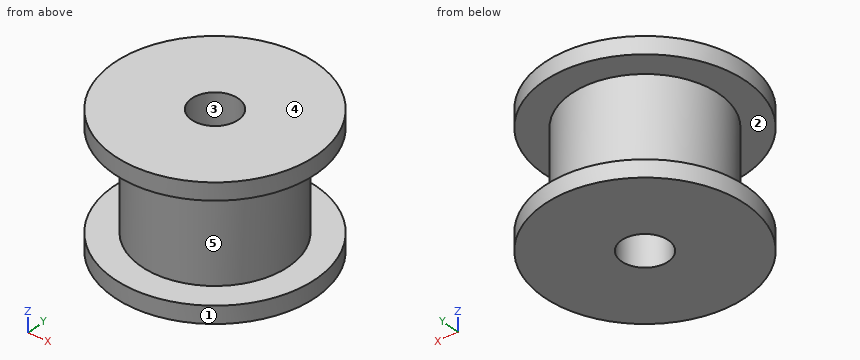
```python
from build123d import *

# Parameters (mm, degrees)
SKETCH_1_R          = 6.5
EXTRUDE_1_DEPTH     = 8.5
SKETCH_2_R          = 1.5
CUT_EXTRUDE_1_DEPTH = 10
SKETCH_3_R          = 9
SKETCH_3_R_2        = 4.75
CUT_EXTRUDE_2_DEPTH = 6.3


with BuildPart() as part:
    # 草图1 → 凸台-拉伸1 (new body)
    with BuildSketch(Plane.XY):
        Circle(SKETCH_1_R)
    extrude(amount=EXTRUDE_1_DEPTH)

    # 草图2 → 切除-拉伸1 (cut)
    with BuildSketch(Plane.XY.offset(8.5)):
        Circle(SKETCH_2_R)
    extrude(amount=-CUT_EXTRUDE_1_DEPTH, mode=Mode.SUBTRACT)

    # 草图3 → 切除-拉伸2 (cut)
    with BuildSketch(Plane.XY.offset(7.4)):
        Circle(SKETCH_3_R)
        Circle(SKETCH_3_R_2, mode=Mode.SUBTRACT)
    extrude(amount=-CUT_EXTRUDE_2_DEPTH, mode=Mode.SUBTRACT)


solid = part.part
```
For this review, take the finished solid that the model builds, in its own axes (mm). Face numbers are marked on the shaded views. A direction names the side the tool comes from. Coordinates: 2 decimals unless noted, no trailing zeros. Order: outer loops, then holes, each group sorted by start corner. A loop starts at its lowest first (then second) coordinate and runs counter-clockwise, first axis right, second up. Notation, with made-up numbers: (54.5, 21.5) -> (70.5, 21.5) arc R25 ccw to (70.5, 50.5) -> close; hole circle Ø2 at (36, 65). An arc over 180 degrees is marked (long way). Answer as CSV lines item,"result".
Q1. We need section C-C (z = 6.5). State the section outline as (x, y) points.
Model answer:
outline,"circle Ø9.5 at (0, 0); hole circle Ø3 at (0, 0)"
Q2. Clearance check with flat-ended pins moving along their axes: pin 1 Ø4 at (x, z) = (0, 5) entering from -Y; pin 2 Ø3 at (y, z) = (3.5, 3) entering from +X. State where each tip first meets the part, or that it passes through.
Model answer:
pin 1,"stops at y = -4.75"
pin 2,"stops at x = 4.31"
Q3. Wall thickness on line 1 along Z through (x, y) = (-4.75, 1.75); line 2 along Y through (x, z) = (0, 6.75); line 3 along X through (y, z) = (0.75, 2.5): over which ranges is each line inside the solid? List them lowest first. Write a range as [from, to].
Model answer:
line 1,"z = [0, 1.1], [7.4, 8.5]"
line 2,"y = [-4.75, -1.5], [1.5, 4.75]"
line 3,"x = [-4.69, -1.3], [1.3, 4.69]"
Q4. For the marked faces 1 and 2, list the 3-axis set-ups (+Z, -Z, +X, -X, +Y, -Y) from which the entire face can be reached by the end or side of a thin tool; tool diameter is ignored.
Model answer:
face 1,"+Z, -Z"
face 2,"none"
Q5. We need section A-A (x = 0). State the section outline as (y, z) points, plus the area to 4 significant figures.
Model answer:
outline,"(-6.5, 0) -> (-1.5, 0) -> (-1.5, 8.5) -> (-6.5, 8.5) -> (-6.5, 7.4) -> (-4.75, 7.4) -> (-4.75, 1.1) -> (-6.5, 1.1) -> close; (1.5, 0) -> (6.5, 0) -> (6.5, 1.1) -> (4.75, 1.1) -> (4.75, 7.4) -> (6.5, 7.4) -> (6.5, 8.5) -> (1.5, 8.5) -> close"
area,"62.95 mm2"
Q6. Draft analysis for pull direction Y (two halves, no side actions). For the marked faces 3, 4 and 5, state which applies: released by +Y, released by -Y, zero draft, split by the parting line, or undercut.
Model answer:
face 3,"undercut"
face 4,"zero draft"
face 5,"split by the parting line"
Q7. We need section D-D (x = -3.5). State the section outline as (y, z) points, plus the area to 3 significant figures.
Model answer:
outline,"(-5.48, 0) -> (5.48, 0) -> (5.48, 1.1) -> (3.21, 1.1) -> (3.21, 7.4) -> (5.48, 7.4) -> (5.48, 8.5) -> (-5.48, 8.5) -> (-5.48, 7.4) -> (-3.21, 7.4) -> (-3.21, 1.1) -> (-5.48, 1.1) -> close"
area,"64.6 mm2"
